Part model, mm, in its own coordinate system. A direction names the side the tool comes from. Give positions to 0.01 mm unless a question says otherwise; leave off trailing zeros. Write each loop counter-clockwise with the first axis right and the second up, starting at its lowest first coordinate (ties: lowest second). Pieces come first, ordered by that corner, then holes.
```python
from build123d import *

# Parameters (mm, degrees)
SKETCH1_R           = 30
BOSS_EXTRUDE1_DEPTH = 47
SKETCH2_R           = 5.5
CUT_EXTRUDE1_DEPTH  = 32
FILLET1_R           = 8
SKETCH2_3_R         = 5.5
CUT_EXTRUDE2_DEPTH  = 35


with BuildPart() as part:
    # Sketch1 → Boss-Extrude1 (new body)
    with BuildSketch(Plane(origin=(0, 0, 0), x_dir=(1, 0, 0), z_dir=(0, 1, 0))):
        Circle(SKETCH1_R)
    extrude(amount=BOSS_EXTRUDE1_DEPTH)

    # Sketch2 → Cut-Extrude1 (cut)
    with BuildSketch(Plane(origin=(0, 47, 0), x_dir=(1, 0, 0), z_dir=(0, 1, 0))):
        with Locations((0, 15.52)):
            Circle(SKETCH2_R)
        with Locations((-13.440714267, 7.76)):
            Circle(SKETCH2_R)
        with Locations((-13.440714267, -7.76)):
            Circle(SKETCH2_R)
        with Locations((0, -15.52)):
            Circle(SKETCH2_R)
        with Locations((13.440714267, -7.76)):
            Circle(SKETCH2_R)
        with Locations((13.440714267, 7.76)):
            Circle(SKETCH2_R)
    extrude(amount=-CUT_EXTRUDE1_DEPTH, mode=Mode.SUBTRACT)

    # Fillet1
    fillet1_edges = [part.edges().sort_by_distance(p)[0] for p in [
        (-30, 0, 0),
    ]]
    fillet(fillet1_edges, radius=FILLET1_R)

    # Sketch2<3> → Cut-Extrude2 (cut)
    with BuildSketch(Plane(origin=(0, 47, 0), x_dir=(1, 0, 0), z_dir=(0, 1, 0))):
        with Locations((0, 15.52)):
            Circle(SKETCH2_3_R)
        with Locations((-13.440714267, 7.76)):
            Circle(SKETCH2_3_R)
        with Locations((-13.440714267, -7.76)):
            Circle(SKETCH2_3_R)
        with Locations((0, -15.52)):
            Circle(SKETCH2_3_R)
        with Locations((13.440714267, -7.76)):
            Circle(SKETCH2_3_R)
        with Locations((13.440714267, 7.76)):
            Circle(SKETCH2_3_R)
    extrude(amount=-CUT_EXTRUDE2_DEPTH, mode=Mode.SUBTRACT)


solid = part.part
```
1) Saw through at B-B, the plane y = 6. Write the cut outline in (x, z).
Answers follow:
outline: circle Ø59.49 at (0, 0)
2) Saw through at A-A, the plane y = 32. Write the cut outline in (x, z), then the cut area to 3 significant figures.
Answers follow:
outline: circle Ø60 at (0, 0); hole circle Ø11 at (-13.44, -7.76); hole circle Ø11 at (-13.44, 7.76); hole circle Ø11 at (0, -15.52); hole circle Ø11 at (0, 15.52); hole circle Ø11 at (13.44, -7.76); hole circle Ø11 at (13.44, 7.76)
area: 2,260 mm2
3) Pin check, flat tips, straight feed: pin 1 Ø12 at (y, z) = (34.5, -15) entering from -X; pin 2 Ø9 at (x, z) = (0, -15.52) entering from +Y; pin 3 Ø1 at (y, z) = (30.5, -12) entering from +X. Stop position of each tip, or through.
Answers follow:
pin 1: stops at x = -28.62
pin 2: stops at y = 12
pin 3: stops at x = 27.71
4) 3-axis set-ups, long thin cutter, end or side, ignore diameter. For faces 1 (the face through (0, 0, 0)), 2 (the face through (13, 12, 8)): which of +Z, -Z, +X, -X, +Y, -Y reach the whole face in a straight line?
Answers follow:
face 1: +Z, -Z, +X, -X, -Y
face 2: +Y
5) Two-plate mould, pull along Z, no slides. Class faces 3 (the face through (2.54, 29.74, 20.4)), 4 (the face through (0, 47, 0)), 5 (the face through (-29.97, 27.23, -1.32)): +Z half, -Z half, draft (parallel to the pull), parting line (faces both ways), or undercut.
Answers follow:
face 3: undercut
face 4: draft
face 5: parting line
6) Wall check: L1, parallel to Z at x = 0, y = 34; L2, parallel to X at y = 45, z = 9.5; L3, parallel to Z at x = -1, y = 34.5. Give the ranges that are in metal, low to high.
Answers follow:
L1: z = -30 to -21.02, -10.02 to 10.02, 21.02 to 30
L2: x = -28.46 to -18.66, -8.22 to 8.22, 18.66 to 28.46
L3: z = -29.98 to -20.93, -10.11 to 10.11, 20.93 to 29.98
